Drawing for the job (mm, zero at the part's lowest x, y, z). Round coordinates to 2 decimals unless told otherwise and drop trailing zeros. Loops run counter-clockwise (first coordinate to the right, second up) from the corner with the lowest first, then second, coordinate; pieces in that order, holes last. Notation, with made-up numbers: M -23.5,78 L -15.5,78 A13 ccw -15.5,100 Z; hole C 13,35 d2. An arc over 180 degrees is marked long. Use a Markdown table: item, result. Add a question column.
Q1. Pin check, flat tips, straight feed: pin 1 (0.8 mm diameter, centred on y = 43.5, z = 1, fed in from +X); pin 2 (0.8 mm diameter, centred on x = 48, z = 1, fed in from +Y). Stop position of each tip, or through.
Q2. Probe line 1 (X direction, y = 8, z = 1.75); line 2 (X direction, y = 55, z = 1.2); line 3 (X direction, y = 9.5, z = 1.05). List the from-to ranges inside material, lowest first. Write a range as from..to.
Q3. Cut at C-C (z = 1.1). Give the cut face in (x, y).
Q4. Cut at D-D (x = 8). Give the cut face in (y, z), plus the area to 3 significant figures.
Q5. Cut at A-A (x = 55). Give the cut face in (y, z), plus the area to 4 significant figures.
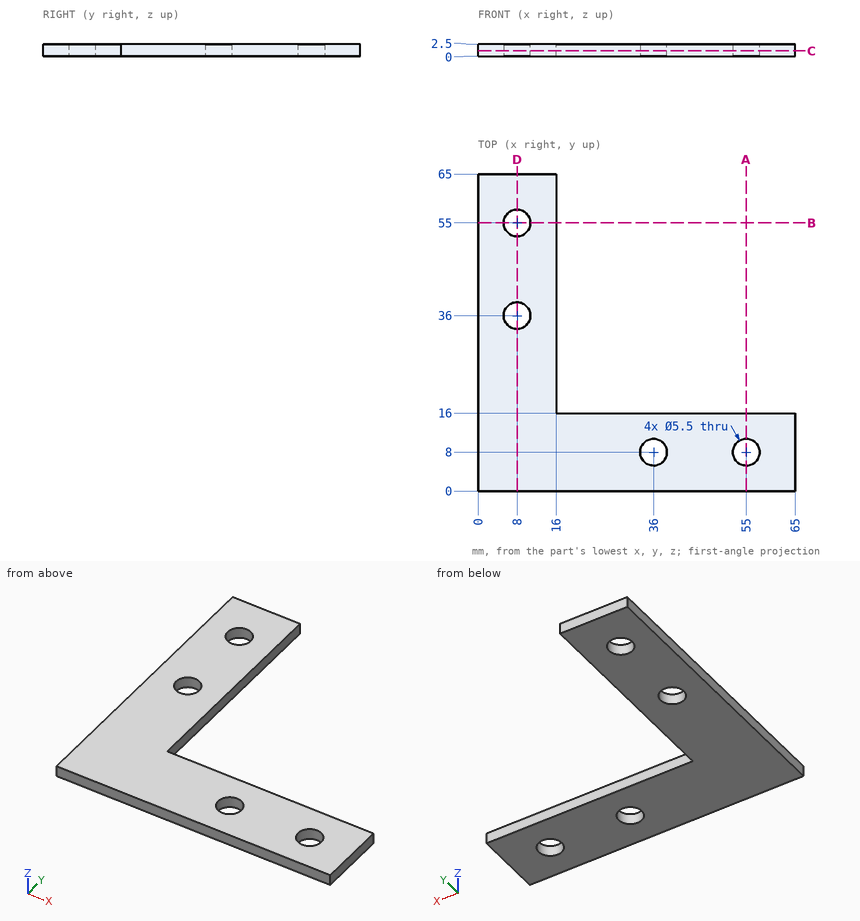
Checked values:
| question | item | result |
|---|---|---|
| 1 | pin 1 | stops at x = 16 |
| 1 | pin 2 | stops at y = 16 |
| 2 | line 1 | x = 0..33.25, 38.75..52.25, 57.75..65 |
| 2 | line 2 | x = 0..5.25, 10.75..16 |
| 2 | line 3 | x = 0..33.7, 38.3..52.7, 57.3..65 |
| 3 | outline | M 0,0 L 65,0 L 65,16 L 16,16 L 16,65 L 0,65 Z; hole C 8,36 d5.5; hole C 8,55 d5.5; hole C 36,8 d5.5; hole C 55,8 d5.5 |
| 4 | outline | M 0,0 L 33.25,0 L 33.25,2.5 L 0,2.5 Z; M 38.75,0 L 52.25,0 L 52.25,2.5 L 38.75,2.5 Z; M 57.75,0 L 65,0 L 65,2.5 L 57.75,2.5 Z |
| 4 | area | 135 mm^2 |
| 5 | outline | M 0,0 L 5.25,0 L 5.25,2.5 L 0,2.5 Z; M 10.75,0 L 16,0 L 16,2.5 L 10.75,2.5 Z |
| 5 | area | 26.25 mm^2 |
